Check sheet for the modelled part. Datum: model origin and axes. Units: mm. Coordinates: 2 decimals unless noted, no trailing zeros. Loops run counter-clockwise (first coordinate to the right, second up) from the corner with the lowest first, then second, coordinate; pieces in that order, holes last. Notation, with made-up numbers: (30, 22) -> (78, 22) arc R16 ccw to (78, 53) -> close; hole circle Ø11 at (-8.75, 84). An arc over 180 degrees is marked (long way). Use one line per item in the form item = value.
from build123d import *

# Parameters (mm, degrees)
SKETCH1_W           = 88.9
SKETCH1_H           = 15.748
BOSS_EXTRUDE1_DEPTH = 12.7
FILLET1_R           = 7.62
SKETCH2_R           = 2.54
CUT_EXTRUDE1_DEPTH  = 2.54
SKETCH3_R           = 2.54
CUT_EXTRUDE2_DEPTH  = 7.62
SKETCH4_R           = 1.016
CUT_EXTRUDE3_DEPTH  = 5.08


with BuildPart() as part:
    # Sketch1 → Boss-Extrude1 (new body)
    with BuildSketch(Plane(origin=(0, 0, 0), x_dir=(1, 0, 0), z_dir=(0, 1, 0))):
        with Locations((12.118156109, 3.2385)):
            Rectangle(SKETCH1_W, SKETCH1_H)
    extrude(amount=BOSS_EXTRUDE1_DEPTH)

    # Fillet1
    fillet1_edges = [part.edges().sort_by_distance(p)[0] for p in [
        (-32.331843891, 6.35, -11.1125),
        (56.568156109, 6.35, -11.1125),
        (56.568156109, 6.35, 4.6355),
        (-32.331843891, 6.35, 4.6355),
    ]]
    fillet(fillet1_edges, radius=FILLET1_R)

    # Sketch2 → Cut-Extrude1 (cut)
    with BuildSketch(Plane(origin=(0, 12.7, 0), x_dir=(1, 0, 0), z_dir=(0, 1, 0))):
        with Locations((-26.428712343, 3.2385)):
            Circle(SKETCH2_R)
    extrude(amount=-CUT_EXTRUDE1_DEPTH, mode=Mode.SUBTRACT)

    # Sketch3 → Cut-Extrude2 (cut)
    with BuildSketch(Plane.XZ):
        with Locations((-26.428712343, -3.2385)):
            Circle(SKETCH3_R)
    extrude(amount=-CUT_EXTRUDE2_DEPTH, mode=Mode.SUBTRACT)

    # Sketch4 → Cut-Extrude3 (cut)
    with BuildSketch(Plane(origin=(0, 10.16, 0), x_dir=(1, 0, 0), z_dir=(0, 1, 0))):
        with Locations((-26.428712343, 3.2385)):
            Circle(SKETCH4_R)
    extrude(amount=-CUT_EXTRUDE3_DEPTH, mode=Mode.SUBTRACT)


solid = part.part
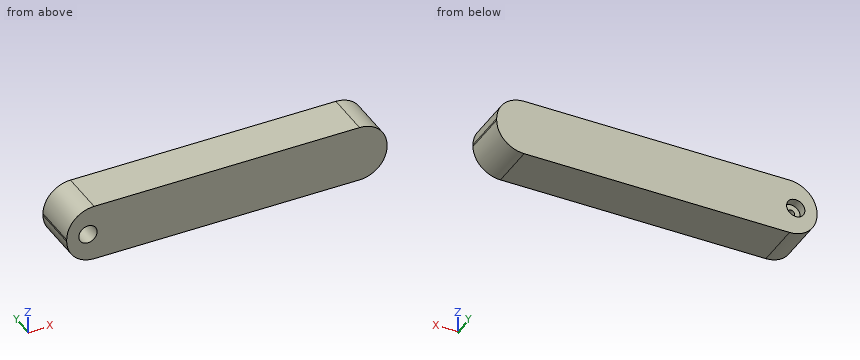
(1) Section check C-C, the plane z = -9.25. Record the boundary of the cut face in (x, y).
Established:
outline = (-29.7, 0) -> (53.94, 0) -> (53.94, 12.7) -> (-29.7, 12.7) -> close
(2) Section check A-A, the plane y = 6.5. Record the boundary of the cut face in (x, z).
Established:
outline = (-32.33, -3.49) arc R7.62 ccw to (-24.71, -11.11) -> (48.95, -11.11) arc R7.62 ccw to (56.57, -3.49) -> (56.57, -2.98) arc R7.62 ccw to (48.95, 4.64) -> (-24.71, 4.64) arc R7.62 ccw to (-32.33, -2.98) -> close; hole circle Ø5.08 at (-26.43, -3.24)
(3) Scan lines: line 1 along X through (y, z) = (1.25, -3.25); line 2 along Z through (x, y) = (-27, 6.25); line 3 along X through (y, z) = (1.25, -5). Record each from-to range of solid material in increasing order.
Established:
line_1 = -32.33 to -28.97, -23.89 to 56.57
line_2 = -10.76 to -5.71, -0.76 to 4.28
line_3 = -32.18 to -28.26, -24.6 to 56.42
(4) Section check B-B, the plane z = 0.5. Record the boundary of the cut face in (x, y), plus the area to 3 significant figures.
Established:
outline = (-31.49, 0) -> (55.72, 0) -> (55.72, 12.7) -> (-31.49, 12.7) -> close
area = 1,110 mm²
(5) Go/stop test with flat-tipped pins: P1, Ø4, axis at x = -26.43, z = -3.24, coming from the +Y side; P2, Ø1, axis at x = 1, z = -8, coming from the -Y side; P3, Ø5, axis at y = 3, z = -9, coming from the -X side. Record where each tip stops, or that it passes through.
Established:
P1 = 10.16
P2 = 0
P3 = -31.71
